Geometry: final body of the model. Coordinates: model frame, mm. Face numbers are marked on the shaded views. A direction names the side the tool comes from. Coordinates: 2 decimals unless noted, no trailing zeros. Write each loop counter-clockwise with the first axis right and the second up, starting at its lowest first coordinate (ties: lowest second). Pieces come first, ordered by that corner, then holes. Notation, with made-up numbers: (34, -28) - (53, -28) arc R16 cw to (53, -11) - close; hole circle Ø7 at (43.25, -34). An arc over 180 degrees is marked (long way). Put each result on its own line as item: value.
Autodesk Inventor part; units mm, degrees
ref_plane "XZ Plane" through (0, 0, 0) normal (0, 1, 0) x (-1, 0, 0)
ref_plane "XY Plane" through (0, 0, 0) normal (0, 0, 1) x (1, 0, 0)
sketch "Náčrt1" plane through (0, 0, 0) normal (0, 0, 1) x (1, 0, 0)
  line L0 (0, 0) -> (80, 0)
  line L1 (80, 0) -> (80, 40)
  line L2 (80, 40) -> (0, 40)
  line L3 (0, 40) -> (0, 0)
  circle A0 centre (16, 20) radius 8
  circle A1 centre (64, 20) radius 8
  dimension "d0" = 80
  dimension "d1" = 40
  dimension "d2" = 16
  dimension "d3" = 16
extrude "Vysunutí1" add sketch "Náčrt1" against normal blind 14
ref_plane "Pracovní rovina1" through (40, 0, 0) normal (1, 0, 0) x (0, 1, 0)
sketch "Náčrt2" plane through (40, 0, 0) normal (1, 0, 0) x (0, 1, 0)
  line L0 (0, -14) -> (40, -14)
  line L1 (40, -14) -> (69, -14)
  line L2 (40, 0) -> (0, 0)
  circle A0 centre (65.4628, 4) radius 9
  arc A1 (69, -14) -> (69, 22) centre (65.4628, 4) ccw
  line L3 (69, 22) -> (30, 22)
  line L4 (30, 22) -> (0, 0)
  line L5 (0, 0) -> (0, -14)
  line L6 (0, -14) -> (40, -14)
  dimension "d7" = 29
  dimension "d9" = 18
  dimension "d10" = 36
  dimension "d11" = 18.3443
  dimension "d12" = 39
extrude "Vysunutí2" add sketch "Náčrt2" along normal mid plane 14
properties part number "14"
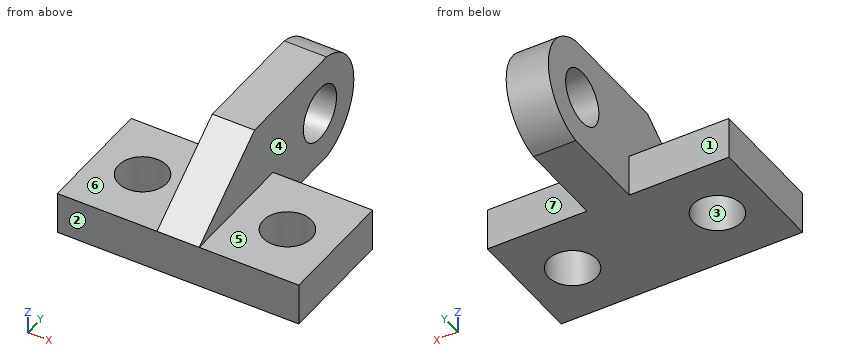
1. Section query D-D (x = 35). Return loops of the section in (y, z), then the cut area to 3 significant figures.
Answer below:
outline: (0, -14) - (69, -14) arc R18.34 ccw to (69, 22) - (30, 22) - (0, 0) - close; hole circle Ø18 at (65.46, 4)
area: 2,300 mm²
2. Ray query, probe 1 along X at (y, z) = (15.5, -3); probe 2 along Y at (x, z) = (64, -4.25); probe 3 along Z at (x, y) = (32, 39.5). Return the intervals inside material, ascending. Write a range as from..to.
Answer below:
probe 1: x = 0..9.39, 22.61..57.39, 70.61..80
probe 2: y = 0..12, 28..40
probe 3: z = -14..0
3. Mould query, pull axis Y, two halves, no side actions, for the marked faces 1, 2, 3 and 4. Classes: +Y half, -Y half, draft (parallel to the pull), parting line (faces both ways), or undercut.
Answer below:
face 1: +Y half
face 2: -Y half
face 3: undercut
face 4: draft
4. Pin query (flat end, axial travel): pin 1 Ø9.5 at (x, y) = (64, 20) entering from -Z; pin 2 Ø7 at (x, z) = (14, -8) entering from +Y; pin 3 Ø18 at (y, z) = (61, 0) entering from -X; pin 4 Ø3 at (x, y) = (26, 41) entering from +Z. Return the tip coordinate at first contact, or that it passes through.
Answer below:
pin 1: passes through
pin 2: stops at y = 40
pin 3: stops at x = 33
pin 4: stops at z = 0
5. Section query C-C (y = 36). Return loops of the section in (x, z), then the cut area to 3 significant figures.
Answer below:
outline: (0, -14) - (80, -14) - (80, 0) - (47, 0) - (47, 22) - (33, 22) - (33, 0) - (0, 0) - close
area: 1,430 mm²
6. Set-up query: the marked faces 5, 6 and 7. Return all of +Z, -Z, +X, -X, +Y, -Y with unobstructed straight access to the full face (end or side cutting, diameter ignored); none if empty.
Answer below:
face 5: +Z, +X, +Y, -Y
face 6: +Z, -X, +Y, -Y
face 7: +Z, -Z, +X, +Y
7. Section query A-A (x = 64). Return loops of the section in (y, z), then the cut area to 3 significant figures.
Answer below:
outline: (0, -14) - (12, -14) - (12, 0) - (0, 0) - close; (28, -14) - (40, -14) - (40, 0) - (28, 0) - close
area: 336 mm²
8. Section query B-B (z = -4). Return loops of the section in (x, y).
Answer below:
outline: (0, 0) - (80, 0) - (80, 40) - (47, 40) - (47, 61.34) - (33, 61.34) - (33, 40) - (0, 40) - close; (33, 69.59) - (47, 69.59) - (47, 81.97) - (33, 81.97) - close; hole circle Ø16 at (16, 20); hole circle Ø16 at (64, 20)
